from build123d import *

# Parameters (mm, degrees)
BOSS_EXTRU_1_DEPTH                            = 22.5
TROU_POUR_TARAUDAGE_POUR_TROU_TARAUD_M3_D     = 2.5
TROU_POUR_TARAUDAGE_POUR_TROU_TARAUD_M3_DEPTH = 5
TROU_POUR_TARAUDAGE_POUR_TROU_TARAUD_M3_TIP   = 0.751075774


with BuildPart() as part:
    # Esquisse1 → Boss.-Extru.1 (new body, symmetric)
    with BuildSketch(Plane.XY):
        Polygon((6.5, -5), (13.5, -5), (13.5, 5), (-13.5, 5), (-13.5, -5), (-6.5, -5), (-6.5, -3.5), (-5.5, -3.5), (-5.5, -2.6), (-6.5, -2.6), (-6.5, 0), (6.5, 0), (6.5, -2.6), (5.5, -2.6), (5.5, -3.5), (6.5, -3.5), align=None)
    extrude(amount=BOSS_EXTRU_1_DEPTH, both=True)

    # Trou pour taraudage pour trou taraudé M3x0.51
    with Locations(Plane(origin=(0, 5, 0), x_dir=(1, 0, 0), z_dir=(0, 1, 0))):
        with Locations((-10, 10), (-10, -10), (10, -10), (10, 10)):
            Hole(TROU_POUR_TARAUDAGE_POUR_TROU_TARAUD_M3_D / 2, depth=TROU_POUR_TARAUDAGE_POUR_TROU_TARAUD_M3_DEPTH)
            with Locations((0, 0, -(TROU_POUR_TARAUDAGE_POUR_TROU_TARAUD_M3_DEPTH + TROU_POUR_TARAUDAGE_POUR_TROU_TARAUD_M3_TIP / 2))):  # 118° drill point
                Cone(0, TROU_POUR_TARAUDAGE_POUR_TROU_TARAUD_M3_D / 2, TROU_POUR_TARAUDAGE_POUR_TROU_TARAUD_M3_TIP, mode=Mode.SUBTRACT)


solid = part.part
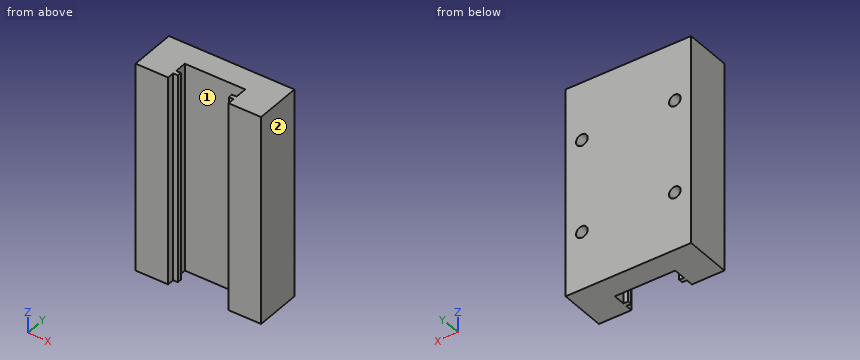
Here's how the part is built. I have some questions about the finished solid (model axes, mm). Face numbers are marked on the shaded views. A direction names the side the tool comes from. Give positions to 0.01 mm unless a question says otherwise; leave off trailing zeros. Order: outer loops, then holes, each group sorted by start corner. A loop starts at its lowest first (then second) coordinate and runs counter-clockwise, first axis right, second up. Notation, with made-up numbers: (33, 50.25) -> (53, 50.25) arc R13 ccw to (53, 72.25) -> close; hole circle Ø7 at (89, 13). An arc over 180 degrees is marked (long way). Use a Markdown table: item, result. Add a question column.
Item 1: For the marked faces 1 and 2, which set-ups out of +Z, -Z, +X, -X, +Y, -Y let a thin tool reach every point of the face, with its end or its side?
Item 2: Will these pins go through, and if not, where does the flat tip stop? pin 1 (2 mm diameter, centred on x = -10, z = -10, fed in from +Y); pin 2 (1.5 mm diameter, centred on x = -10, z = 10, fed in from +Y).
Item 3: Imagine slicing it at A-A on y = 3.5. Please give me the cut outline in (x, z).
Item 4: I need wall thicknesses on line 1 (Z direction, x = -10, y = 2.4); line 2 (X direction, y = 3, z = 10); line 3 (X direction, y = -3.75, z = 12). Which ranges of each line are inside material? Lowest first, please.
Item 5: Imagine slicing it at C-C on x = 4.5. Please give me the cut outline in (y, z), plus the area to 3 significant figures.
Item 6: Imagine slicing it at B-B on z = -6.5. Please give me the cut outline in (x, y), plus the area to 3 significant figures.
Data:
| question | item | result |
|---|---|---|
| 1 | face 1 | +Z, -Z |
| 1 | face 2 | +Z, -Z, +X, +Y, -Y |
| 2 | pin 1 | stops at y = -0.15 |
| 2 | pin 2 | stops at y = -0.3 |
| 3 | outline | (-13.5, -22.5) -> (13.5, -22.5) -> (13.5, 22.5) -> (-13.5, 22.5) -> close; hole circle Ø2.5 at (-10, -10); hole circle Ø2.5 at (-10, 10); hole circle Ø2.5 at (10, -10); hole circle Ø2.5 at (10, 10) |
| 4 | line 1 | z = -22.5 to -11.25, -8.75 to 8.75, 11.25 to 22.5 |
| 4 | line 2 | x = -13.5 to -11.25, -8.75 to 8.75, 11.25 to 13.5 |
| 4 | line 3 | x = -13.5 to -6.5, 6.5 to 13.5 |
| 5 | outline | (0, -22.5) -> (5, -22.5) -> (5, 22.5) -> (0, 22.5) -> close |
| 5 | area | 225 mm² |
| 6 | outline | (-13.5, -5) -> (-6.5, -5) -> (-6.5, -3.5) -> (-5.5, -3.5) -> (-5.5, -2.6) -> (-6.5, -2.6) -> (-6.5, 0) -> (6.5, 0) -> (6.5, -2.6) -> (5.5, -2.6) -> (5.5, -3.5) -> (6.5, -3.5) -> (6.5, -5) -> (13.5, -5) -> (13.5, 5) -> (-13.5, 5) -> close |
| 6 | area | 207 mm² |
